Here's the drawing with two shaded views (mm, measured from the low corner). I have some questions. A direction names the side the tool comes from. Round coordinates to 2 decimals unless told otherwise and drop trailing zeros. Order: outer loops, then holes, each group sorted by start corner. A loop starts at its lowest first (then second) coordinate and runs counter-clockwise, first axis right, second up.
Q1. If we section it at A-A (y = 13): Please give me the cut outline in (x, z) (1 decimal).
Q2. Will these pins go through, and if not, where does the flat tip stop? P1, Ø1.8, axis at y = 14, z = 2, coming from the -X side (1 decimal); P2, Ø3, axis at x = 44.5, y = 10.5, coming from the +Z side; P3, Ø1.8, axis at x = 4.5, y = 8.5, coming from the +Z side.
Q3. We'd pull the mould along Y, two halves only. Please class the marked faces 1, 2, 3 and 4: pulls with the +Y half, pulls with the -Y half, needs draft (parallel to the pull), parting line crosses it, or undercut.
Q4. If we section it at C-C (x = 11.5): Please give me the cut outline in (y, z).
Q5. If we section it at D-D (y = 6.25): Please give me the cut outline in (x, z) (1 decimal).
Q6. If we section it at B-B (z = 0.95): Please give me the cut outline in (x, y) (1 decimal).
Q7. If I drill on line 1 (X direction, y = 2.5, z = 5.15) (1 decimal); line 2 (X direction, y = 7.75, z = 4.7) (1 decimal); line 3 (Y direction, x = 22.5, z = 2.9), over which ranges is the centre line in solid material (lowest first)?
Q8. For the marked faces 5, 6 and 7, which set-ups out of +Z, -Z, +X, -X, +Y, -Y let a thin tool reach every point of the face, with its end or its side?
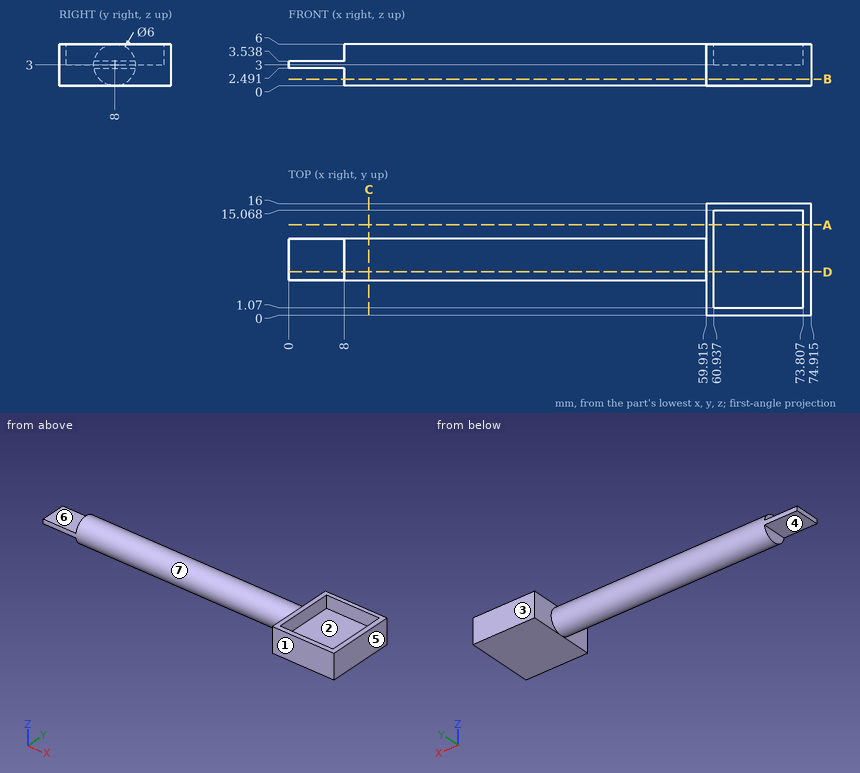
Solution:
1. outline: (59.9, 0) - (74.9, 0) - (74.9, 6) - (73.8, 6) - (73.8, 3) - (60.9, 3) - (60.9, 6) - (59.9, 6) - close
2. P1: stops at x = 59.9
2. P2: stops at z = 5.83
2. P3: stops at z = 3.54
3. face 1: pulls with the -Y half
3. face 2: undercut
3. face 3: pulls with the +Y half
3. face 4: needs draft
4. outline: circle Ø6 at (8, 3)
5. outline: (0, 2.5) - (8, 2.5) - (8, 0.6) - (59.9, 0.6) - (59.9, 0) - (74.9, 0) - (74.9, 6) - (73.8, 6) - (73.8, 3) - (60.9, 3) - (60.9, 6) - (59.9, 6) - (59.9, 5.4) - (8, 5.4) - (8, 3.5) - (0, 3.5) - close
6. outline: (8, 5.8) - (59.9, 5.8) - (59.9, 0) - (74.9, 0) - (74.9, 16) - (59.9, 16) - (59.9, 10.2) - (8, 10.2) - close
7. line 1: x = 59.9 to 60.9, 73.8 to 74.9
7. line 2: x = 8 to 60.9, 73.8 to 74.9
7. line 3: y = 5 to 11
8. face 5: +Z, -Z, +X, +Y, -Y
8. face 6: +Z, -X, +Y, -Y
8. face 7: -X
